For this review, take the finished solid that the model builds, in its own axes (mm). Face numbers are marked on the shaded views. A direction names the side the tool comes from. Round coordinates to 2 decimals unless told otherwise and drop trailing zeros. Order: outer loops, then holes, each group sorted by start corner. A loop starts at its lowest first (then second) coordinate and runs counter-clockwise, first axis right, second up. Notation, with made-up numbers: M 16.25,7.5 L 32.25,7.5 A22 cw 32.25,21.5 Z; hole C -35,-36.75 d3. An arc over 180 degrees is marked long. Answer as a JSON object with one key per item and string values.
from build123d import *
from OCP.BRepFilletAPI import BRepFilletAPI_MakeChamfer

# Parameters (mm, degrees)
BOSS_EXTRUDE1_DEPTH     = 5
BOSS_EXTRUDE1_2_DEPTH   = 5
BOSS_EXTRUDE2_DEPTH     = 33
CUT_EXTRUDE1_DEPTH      = 75.424878233
CUT_EXTRUDE1_DEPTH_BACK = 75.424878233
SKETCH4_W               = 5
SKETCH4_H               = 11.27
BOSS_EXTRUDE3_DEPTH     = 6
CHAMFER1_SIZE           = 10
CHAMFER1_SIZE2          = 3
CUT_EXTRUDE2_DEPTH      = 60.555121526
FILLET1_R               = 3
FILLET2_R               = 3


with BuildPart() as part:
    # Sketch1 → Boss-Extrude1 (new body)
    with BuildSketch(Plane(origin=(0, 0, 0), x_dir=(1, 0, 0), z_dir=(0, 1, 0))):
        Polygon((-18.75, -2.5), (-17.25, 2.5), (-10.25, 2.5), (-8.75, -2.5), align=None)
    extrude(amount=-BOSS_EXTRUDE1_DEPTH)



with BuildPart() as body_2:
    # Sketch1 → Boss-Extrude1 2 (new body)
    with BuildSketch(Plane(origin=(0, 0, 0), x_dir=(1, 0, 0), z_dir=(0, 1, 0))):
        Polygon((17.25, 2.5), (10.25, 2.5), (8.75, -2.5), (18.75, -2.5), align=None)
    extrude(amount=-BOSS_EXTRUDE1_2_DEPTH)


with BuildPart() as part_1:
    add(part.part)

    add(body_2.part)  # Boss-Extrude2 merges body 2
    # Sketch2 → Boss-Extrude2 (add)
    with BuildSketch(Plane(origin=(0, 0, 0), x_dir=(1, 0, 0), z_dir=(0, 1, 0))):
        Polygon((27.5, 2.5), (-27.5, 2.5), (-27.5, -2.5), (-27.5, -37.75), (-22.5, -37.75), (-22.5, -2.5), (22.5, -2.5), (22.5, -37.75), (27.5, -37.75), (27.5, -2.5), align=None)
    extrude(amount=BOSS_EXTRUDE2_DEPTH)

    # Sketch3 → Cut-Extrude1 (cut, two sides: drawn at the far end of the back side and taken through both)
    with BuildSketch(Plane.ZY.offset(27.5).offset(-CUT_EXTRUDE1_DEPTH_BACK)):
        with BuildLine():
            Line((6.265950561, 19.5), (28.984049439, 19.5))
            ThreePointArc((28.984049439, 19.5), (31.984049439, 16.5), (28.984049439, 13.5))
            Line((28.984049439, 13.5), (6.265950561, 13.5))
            ThreePointArc((6.265950561, 13.5), (3.265950561, 16.5), (6.265950561, 19.5))
        make_face()
    extrude(amount=CUT_EXTRUDE1_DEPTH + CUT_EXTRUDE1_DEPTH_BACK, mode=Mode.SUBTRACT)

    # Sketch4 → Boss-Extrude3 (add)
    with BuildSketch(Plane.XY.offset(37.75)):
        with Locations((25, 5.635)):
            Rectangle(SKETCH4_W, SKETCH4_H)
        with Locations((-25, 5.635)):
            Rectangle(SKETCH4_W, SKETCH4_H)
    extrude(amount=BOSS_EXTRUDE3_DEPTH)

    # Chamfer1: one chamfer whose edges measure the first distance from different faces: ONE call of the kernel's chamfer builder (chamfer() names one face for all edges)
    chamfer1_edges_1 = [part_1.edges().sort_by_distance(p)[0] for p in [
        (-25, 33, 37.75),
    ]]
    chamfer1_side_1 = [part_1.faces().sort_by_distance(p)[0] for p in [
        (-25, 22.135, 37.75),
    ]]
    chamfer1_edges_2 = [part_1.edges().sort_by_distance(p)[0] for p in [
        (25, 33, 37.75),
    ]]
    chamfer1_side_2 = [part_1.faces().sort_by_distance(p)[0] for p in [
        (25, 22.135, 37.75),
    ]]
    chamfer1 = BRepFilletAPI_MakeChamfer(part_1.part.solid().wrapped)
    for e in chamfer1_edges_1:
        chamfer1.Add(CHAMFER1_SIZE, CHAMFER1_SIZE2, e.wrapped, chamfer1_side_1[0].wrapped)  # the first distance lies on this face
    for e in chamfer1_edges_2:
        chamfer1.Add(CHAMFER1_SIZE, CHAMFER1_SIZE2, e.wrapped, chamfer1_side_2[0].wrapped)  # the first distance lies on this face
    add(Compound.cast(chamfer1.Shape()), mode=Mode.REPLACE)

    # Sketch7 → Cut-Extrude2 (cut, through all)
    with BuildSketch(Plane.XY.offset(2.5)):
        with BuildLine():
            Line((-15, 19.5), (15, 19.5))
            ThreePointArc((15, 19.5), (18, 16.5), (15, 13.5))
            Line((15, 13.5), (-15, 13.5))
            ThreePointArc((-15, 13.5), (-18, 16.5), (-15, 19.5))
        make_face()
    extrude(amount=-CUT_EXTRUDE2_DEPTH, mode=Mode.SUBTRACT)

    # Fillet1
    fillet1_edges = [part_1.edges().sort_by_distance(p)[0] for p in [
        (27.5, 16.5, -2.5),
        (-27.5, 16.5, -2.5),
    ]]
    fillet(fillet1_edges, radius=FILLET1_R)

    # Fillet2
    fillet2_edges = [part_1.edges().sort_by_distance(p)[0] for p in [
        (27.5, 33, 17.625),
        (-27.5, 33, 17.625),
        (0, 33, -2.5),
        (26.621320344, 33, -1.621320344),
        (-26.621320344, 33, -1.621320344),
    ]]
    fillet(fillet2_edges, radius=FILLET2_R)


solid = part_1.part
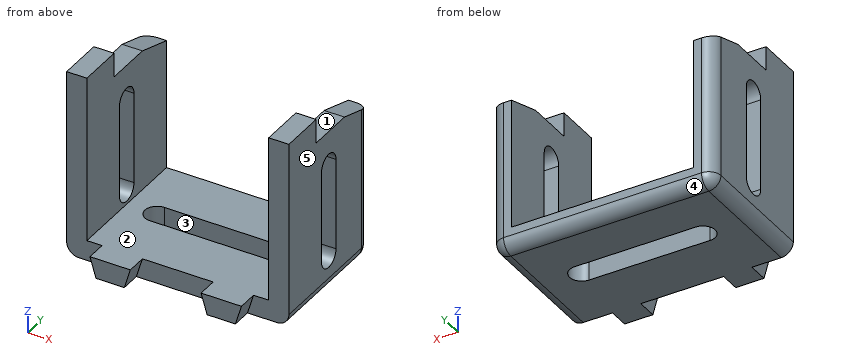
1) Mouldability with a two-part tool opening along Y and no side actions: class the marked faces 3, 4 and 5 as +Y half, -Y half, draft (parallel to the pull), parting line (faces both ways), or undercut.
Geometry check:
{"face 3": "undercut", "face 4": "+Y half", "face 5": "draft"}
2) For L1, parallel to Y at x = 24, z = 10; L2, parallel to X at y = 25.5, z = 7.5; L3, parallel to Y at x = 11.5, z = 1, list the stretches that pass through material, from the lowest coordinate up.
Geometry check:
{"L1": "y = 0 to 13.5, 19.5 to 33", "L2": "x = -27.5 to -22.5, 22.5 to 27.5", "L3": "y = -5 to 13.5, 19.5 to 33"}
3) Machinability: for the marked faces 1 and 2, which of the approach directions +Z, -Z, +X, -X, +Y, -Y give a long, thin tool a straight path to every point of the face, cutting with its end or side? Answer none if there is none.
Geometry check:
{"face 1": "+Z, +X, -X, +Y", "face 2": "+Z, +Y, -Y"}
4) Add section D-D on y = 4.5. State the section outline as (x, z) points, and give its area (3 significant figures).
Geometry check:
{"outline": "M -27.5,0.5 A3 ccw -24.5,-2.5 L 24.5,-2.5 A3 ccw 27.5,0.5 L 27.5,43.75 L 22.5,43.75 L 22.5,2.5 L -22.5,2.5 L -22.5,43.75 L -27.5,43.75 Z", "area": "684 mm²"}
5) Insertion check: P1, Ø4, axis at x = 2.5, z = 0.5, coming from the -Y side; P2, Ø10, axis at y = 15, z = 15.5, coming from the +X side; P3, Ø1.5, axis at x = 26, y = 18, coming from the +Z side; P4, Ø2.5, axis at x = 24, z = 42, coming from the +Y side. Each pin has a flat end and moves straight along its axis. Give the tip position at first contact, or say it passes through.
Geometry check:
{"P1": "stops at y = 0", "P2": "stops at x = 27.5", "P3": "stops at z = 37.75", "P4": "stops at y = 11.27"}
6) Add section C-C on y = 16.5. State the section outline as (x, z) points, and give its area (3 significant figures).
Geometry check:
{"outline": "M -27.5,0.5 A3 ccw -24.5,-2.5 L -18,-2.5 L -18,2.5 L -22.5,2.5 L -22.5,3.27 L -27.5,3.27 Z; M -27.5,31.98 L -22.5,31.98 L -22.5,37.75 L -27.5,37.75 Z; M 18,-2.5 L 24.5,-2.5 A3 ccw 27.5,0.5 L 27.5,3.27 L 22.5,3.27 L 22.5,2.5 L 18,2.5 Z; M 22.5,31.98 L 27.5,31.98 L 27.5,37.75 L 22.5,37.75 Z", "area": "156 mm²"}
7) Add section B-B on x = -13. State the section outline as (y, z) points.
Geometry check:
{"outline": "M -5,-2.5 L 13.5,-2.5 L 13.5,2.5 L -5,2.5 Z; M 19.5,-2.5 L 30,-2.5 A3 ccw 33,0.5 L 33,2.5 L 19.5,2.5 Z"}
8) Add section A-A on z = 26. State the section outline as (x, y) points.
Geometry check:
{"outline": "M -27.5,0 L -22.5,0 L -22.5,13.5 L -27.5,13.5 Z; M -27.5,19.5 L -22.5,19.5 L -22.5,33 L -24.5,33 A3 ccw -27.5,30 Z; M 22.5,0 L 27.5,0 L 27.5,13.5 L 22.5,13.5 Z; M 22.5,19.5 L 27.5,19.5 L 27.5,30 A3 ccw 24.5,33 L 22.5,33 Z"}
